Study the drawing (mm; zero at the part's minimum x, y, z) and answer. Give positions to 0.01 mm unless a question says otherwise; leave off trailing zeros. Loops run counter-clockwise (first coordinate to the right, second up) from the corner with the lowest first, then second, coordinate; pieces in that order, holes last. Notation, with made-up numbers: (21, -3.5) -> (31, -3.5) arc R30 cw to (31, 35.5) -> close; hole circle Ø6 at (-4.75, 49.25). An arc over 180 degrees is marked (long way). One line per question, with ' | ' between items. Start each with the question number.
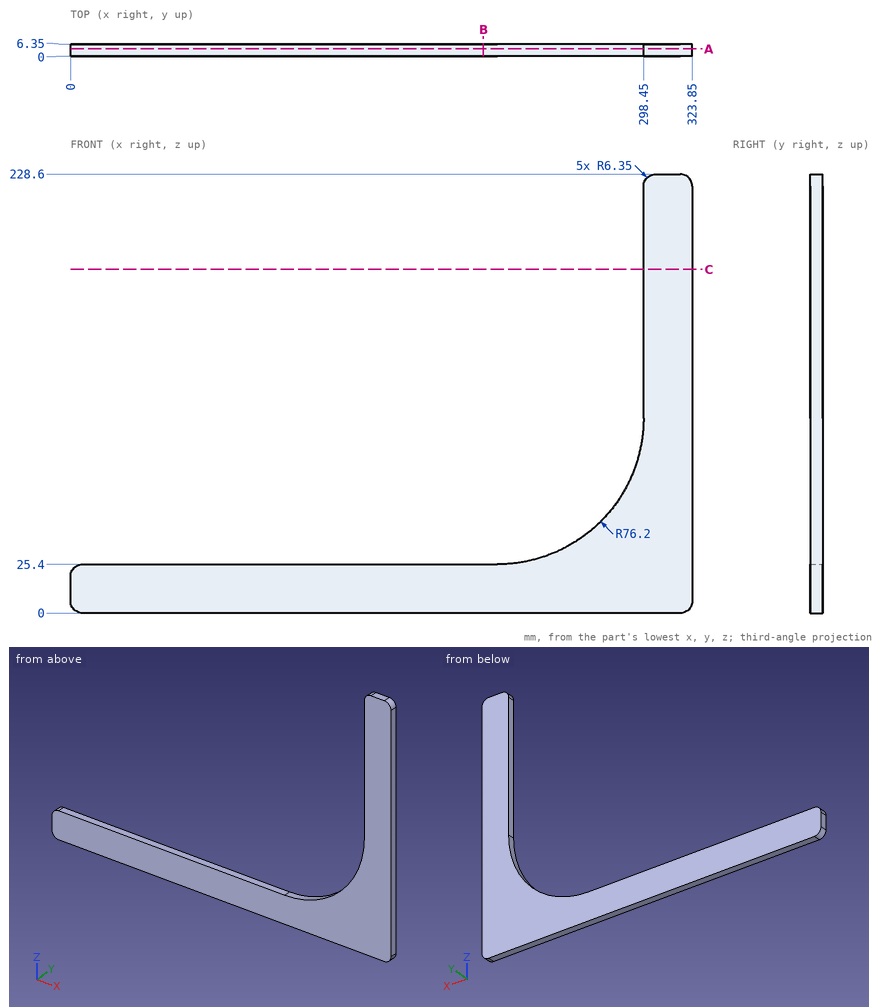
1. The part is cut by section A-A (y = 3.75). Write down the section's boundary in (x, z).
2. Straight lines are drawn through the part: L1, parallel to Z at x = 20, y = 4; L2, parallel to X at y = 2.5, z = 216; L3, parallel to Z at x = 259, y = 1. For each, find the intervals that lie inside material, in ascending order.
3. The part is cut by section C-C (z = 179). Write down the section's boundary in (x, y).
4. Each of these flat-tipped pins is pushed along its axis until it touches: pin 1 Ø1.5 at (y, z) = (2.5, 195) entering from -X; pin 2 Ø1.5 at (y, z) = (2.5, 47) entering from -X; pin 3 Ø2 at (x, y) = (71, 3) entering from +Z. Where does it stop, or does it pass through?
5. The part is cut by section B-B (x = 215). Write down the section's boundary in (y, z), plus the area to 3 significant figures.
Check sheet entries:
1) outline: (0, 6.35) arc R6.35 ccw to (6.35, 0) -> (317.5, 0) arc R6.35 ccw to (323.85, 6.35) -> (323.85, 222.25) arc R6.35 ccw to (317.5, 228.6) -> (304.8, 228.6) arc R6.35 ccw to (298.45, 222.25) -> (298.45, 101.6) arc R76.2 cw to (222.25, 25.4) -> (6.35, 25.4) arc R6.35 ccw to (0, 19.05) -> close
2) L1: z = 0 to 25.4 | L2: x = 298.45 to 323.85 | L3: z = 0 to 34.85
3) outline: (298.45, 0) -> (323.85, 0) -> (323.85, 6.35) -> (298.45, 6.35) -> close
4) pin 1: stops at x = 298.45 | pin 2: stops at x = 274.62 | pin 3: stops at z = 25.4
5) outline: (0, 0) -> (6.35, 0) -> (6.35, 25.4) -> (0, 25.4) -> close | area: 161 mm^2
